from build123d import *

# Parameters (mm, degrees)
SKETCH_R        = 2.2
SKETCH_R_2      = 1.45
PAD_DEPTH       = 33
SKETCH037_R     = 2.2
SKETCH037_R_2   = 1.45
PAD016_DEPTH    = 4.5
SKETCH039_W     = 13.4
SKETCH039_H     = 10
PAD017_DEPTH    = 5
POCKET018_DEPTH = 13.4
SKETCH041_W     = 3.4
SKETCH041_H     = 70.5
POCKET019_DEPTH = 7.1
FILLET006_R     = 1
FILLET007_R     = 4


with BuildPart() as part:
    # Sketch → Pad (new body, symmetric)
    with BuildSketch(Plane.XZ):
        with BuildLine():
            Line((-9.25, -31.677082), (9.25, -31.677082))
            ThreePointArc((9.25, -31.677082), (23.787894, -22.872168), (32.015621, -8))
            Line((-32.015621, -8), (32.015621, -8))
            ThreePointArc((-32.015621, -8), (-23.787894, -22.872168), (-9.25, -31.677082))
        make_face()
        with Locations((24.9, -12.6)):
            Circle(SKETCH_R, mode=Mode.SUBTRACT)
        with Locations((-24.9, -12.6)):
            Circle(SKETCH_R, mode=Mode.SUBTRACT)
        with Locations((0, -12.6)):
            Circle(SKETCH_R_2, mode=Mode.SUBTRACT)
        with BuildLine():
            ThreePointArc((0, -18.243174), (-6.771568, -11.057878), (-16.248592, -13.827105))
            ThreePointArc((-16.248592, -13.827105), (-21.564175, -13.876493), (-18.494342, -18.216307))
            ThreePointArc((-18.494342, -18.216307), (-11.197344, -29.424262), (0, -22.11099))
            ThreePointArc((0, -22.11099), (18.7, -20.177082), (0, -18.243174))
        make_face(mode=Mode.SUBTRACT)
    extrude(amount=PAD_DEPTH, both=True)

    # Sketch037 (on Face13 of Pad) → Pad016 (join)
    with BuildSketch(Plane.XZ.offset(33)):
        with BuildLine():
            ThreePointArc((-32.015621, -8), (-23.787894, -22.872168), (-9.25, -31.677082))
            Line((9.25, -31.677082), (-9.25, -31.677082))
            ThreePointArc((9.25, -31.677082), (23.787894, -22.872168), (32.015621, -8))
            Line((-32.015621, -8), (32.015621, -8))
        make_face()
        with Locations((-24.9, -12.6)):
            Circle(SKETCH037_R, mode=Mode.SUBTRACT)
        with Locations((0, -12.6)):
            Circle(SKETCH037_R_2, mode=Mode.SUBTRACT)
        with Locations((24.9, -12.6)):
            Circle(SKETCH037_R, mode=Mode.SUBTRACT)
    extrude(amount=PAD016_DEPTH)

    # Sketch039 → Pad017 (join)
    with BuildSketch(Plane(origin=(0, 0, -8), x_dir=(-1, 0, 0), z_dir=(0, 0, 1))):
        with Locations((0, 32.5)):
            Rectangle(SKETCH039_W, SKETCH039_H)
    extrude(amount=PAD017_DEPTH)

    # Sketch040 (on Face8 of Pad017) → Pocket018 (cut)
    with BuildSketch(Plane(origin=(6.7, 0, 0), x_dir=(0, 0, 1), z_dir=(1, 0, 0))):
        with BuildLine():
            Line((-6.224874, 30.75), (-4.775126, 30.75))
            Line((-4.775126, 30.75), (-4.262563, 31.262563))
            ThreePointArc((-4.262563, 31.262563), (-5.5, 34.25), (-6.737437, 31.262563))
            Line((-6.224874, 30.75), (-6.737437, 31.262563))
        make_face()
    extrude(amount=-POCKET018_DEPTH, mode=Mode.SUBTRACT)

    # Sketch041 (on Face22 of Pocket018) → Pocket019 (cut)
    with BuildSketch(Plane(origin=(0, 0, -3), x_dir=(-1, 0, 0), z_dir=(0, 0, 1))):
        with Locations((0, 2.25)):
            Rectangle(SKETCH041_W, SKETCH041_H)
    extrude(amount=-POCKET019_DEPTH, mode=Mode.SUBTRACT)

    # Fillet006
    fillet006_edges = [part.edges().sort_by_distance(p)[0] for p in [
        (6.7, -32.5, -3),
        (1.7, -32.5, -3),
        (-1.7, -32.5, -3),
        (-6.7, -32.5, -3),
    ]]
    fillet(fillet006_edges, radius=FILLET006_R)

    # Fillet007
    fillet007_edges = [part.edges().sort_by_distance(p)[0] for p in [
        (-4.2, -27.5, -8),
        (4.2, -27.5, -8),
    ]]
    fillet(fillet007_edges, radius=FILLET007_R)


solid = part.part
Work out the finished part from the listing and answer in its coordinate system (mm). A direction names the side the tool comes from. Give positions to 0.01 mm unless a question says otherwise; leave off trailing zeros. Loops run counter-clockwise (first coordinate to the right, second up) from the corner with the lowest first, then second, coordinate; pieces in that order, holes last. Notation, with made-up numbers: (15.5, 72) - (70.5, 72) arc R24 cw to (70.5, 107) - close; hole circle Ø7 at (-19.75, 39). An arc over 180 degrees is marked (long way). Answer in a Markdown table with one row per item.
(1) Section D-D (x = -21) is taken. Give the vertices of the cut face in (y, z).
Results list:
| item | result |
|---|---|
| outline | (-37.5, -25.46) - (33, -25.46) - (33, -17.38) - (-33, -17.38) - (-33, -13.11) - (33, -13.11) - (33, -8) - (-37.5, -8) - close |
(2) For a pull along X with two mould halves and no side action, classify faces 1 (the face through (-11.4, -0.46, -29.38)), 2 (the face through (-4.235, -26.297, -6.859)), 3 (the face through (-1.7, -7, -9)), 4 (the face through (-23.95, -1.76, -22.7)) as pulls with the +X half, pulls with the -X half, needs draft (parallel to the pull), parting line crosses it, or undercut.
Results list:
| item | result |
|---|---|
| face 1 | undercut |
| face 2 | needs draft |
| face 3 | undercut |
| face 4 | pulls with the -X half |
(3) Consider L1, parallel to X at y = -31.5, z = -7; L2, parallel to X at y = -1.5, z = -28; L3, parallel to Y at x = -16, z = -14. Determine where each line is inside the solid, lowest interval first. Write a range as [from, to].
Results list:
| item | result |
|---|---|
| L1 | x = [-6.7, -1.7], [1.7, 6.7] |
| L2 | x = [-17.46, -14.55], [-3.95, 3.95], [14.55, 17.46] |
| L3 | y = [-37.5, -33] |
(4) A tool of negligible diameter and unlimited length cuts with its end or side. For faces 5 (the face through (1.7, -7, -9)), 6 (the face through (-21.521, -0.462, -13.796)), 7 (the face through (6.7, -32, -7.4)), from which of +Z, -Z, +X, -X, +Y, -Y can it reach the whole face along a straight path? Write none if from no direction.
Results list:
| item | result |
|---|---|
| face 5 | +Z, +Y, -Y |
| face 6 | +Y |
| face 7 | +Z, +X, +Y, -Y |
(5) Flat-ended cylindrical pins translate along their axes: pin 1 Ø10 at (x, y) = (21.5, 14.5) entering from +Z; pin 2 Ø4 at (y, z) = (-32.5, -5.5) entering from +X; pin 3 Ø1.5 at (y, z) = (-8, -17.5) entering from -X. Find the tip coordinate at first contact, or state that the pin passes through.
Results list:
| item | result |
|---|---|
| pin 1 | stops at z = -8 |
| pin 2 | stops at x = 6.7 |
| pin 3 | stops at x = -28.43 |
(6) Section C-C (z = -21) is taken. Give the vertices of the cut face in (x, y), and give its area (3 significant figures).
Results list:
| item | result |
|---|---|
| outline | (-25.46, -37.5) - (25.46, -37.5) - (25.46, 33) - (18.66, 33) - (18.66, -33) - (-18.66, -33) - (-18.66, 33) - (-25.46, 33) - close |
| area | 1,130 mm² |
(7) Section A-A (x = 24.9) is taken. Give the vertices of the cut face in (y, z), and give its area (3 significant figures).
Results list:
| item | result |
|---|---|
| outline | (-37.5, -21.66) - (33, -21.66) - (33, -14.8) - (-37.5, -14.8) - close; (-37.5, -10.4) - (33, -10.4) - (33, -8) - (-37.5, -8) - close |
| area | 653 mm² |
